Autodesk Inventor part; units mm, degrees
ref_plane "YZ Plane" through (0, 0, 0) normal (1, 0, 0) x (0, 1, 0)
ref_plane "XZ Plane" through (0, 0, 0) normal (0, 1, 0) x (-1, 0, 0)
ref_plane "XY Plane" through (0, 0, 0) normal (0, 0, 1) x (1, 0, 0)
sketch "Sketch1" plane through (0, 0, 0) normal (0, 1, 0) x (-1, 0, 0)
  line L0 (20.5, 16.2) -> (-20.5, 16.2)
  line L1 (-20.5, 16.2) -> (-20.5, -16.2)
  line L2 (-20.5, -16.2) -> (20.5, -16.2)
  line L3 (20.5, -16.2) -> (20.5, 16.2)
  point P0 (0, 0)
  dimension "d0" = 41
  dimension "d1" = 32.4
extrude "Extrusion1" add sketch "Sketch1" along normal blind 3
sketch "Sketch3" plane through (0, 3, 0) normal (0, 1, 0) x (1, 0, 0)
  line L0 (-20.5, -16.2) -> (20.5, -16.2)
  line L1 (-20.5, 16.2) -> (-20.5, -16.2)
  line L2 (20.5, -16.2) -> (-20.5, -16.2)
  line L3 (-20.5, -16.2) -> (-20.5, -13.2)
  line L4 (-20.5, -13.2) -> (20.5, -13.2)
  line L5 (20.5, -13.2) -> (20.5, -16.2)
  line L6 (20.5, 16.2) -> (-20.5, 16.2)
  line L7 (20.5, 16.2) -> (-20.5, 16.2)
  line L8 (-20.5, 16.2) -> (-20.5, 13.2)
  line L9 (-20.5, 13.2) -> (20.5, 13.2)
  line L10 (20.5, 13.2) -> (20.5, 16.2)
  point P0 (0, 0)
  dimension "d8" = 3
  dimension "d9" = 3
extrude "Extrusion3" add sketch "Sketch3" along normal blind 25.4
sketch "Sketch4" plane through (20.5, 0, -16.2) normal (0, 0, -1) x (-1, 0, 0)
  line L0 (41, 3) -> (0, 3)
  line L1 (0, 28.4) -> (41, 28.4)
  line L2 (0, 3) -> (21.5, 3)
  line L3 (21.5, 3) -> (21.5, 28.4)
  line L4 (21.5, 28.4) -> (0, 28.4)
  line L5 (0, 28.4) -> (0, 3)
  point P0 (20.5, 0)
  dimension "d12" = 21.5
extrude "Extrusion4" cut sketch "Sketch4" against normal blind 3
sketch "Sketch5" plane through (-20.5, 0, 16.2) normal (0, 0, 1) x (1, 0, 0)
  line L0 (41, 28.4) -> (0, 28.4)
  line L1 (19.5, 3) -> (41, 3)
  line L2 (0, 28.4) -> (21.5, 28.4)
  line L3 (21.5, 28.4) -> (21.5, 3)
  line L4 (21.5, 3) -> (0, 3)
  line L5 (0, 3) -> (0, 28.4)
  point P0 (20.5, 0)
  dimension "d15" = 21.5
extrude "Extrusion5" cut sketch "Sketch5" against normal blind 3
sketch "Sketch6" plane through (0, 3, 0) normal (0, 1, 0) x (1, 0, 0)
  circle A0 centre (13, 0) radius 4.25
  circle A1 centre (-13, 0) radius 4.25
  line L0 (20.5, -13.2) -> (20.5, 16.2)
  line L1 (-20.5, 13.2) -> (-20.5, -16.2)
  point P0 (0, 0)
  dimension "d20" = 8.5
  dimension "d21" = 8.5
  dimension "d54" = 7.5
  dimension "d65" = 26
  dimension "d66" = 7.5
extrude "Extrusion6" add sketch "Sketch6" along normal blind 3
sketch "Sketch7" plane through (0, 0, 0) normal (0, -1, 0) x (1, 0, 0)
  circle A0 centre (-13, 0) radius 4.25
  circle A1 centre (-13, 0) radius 2
  circle A2 centre (13, 0) radius 4.25
  circle A3 centre (13, 0) radius 2
  point P0 (0, 0)
  dimension "d24" = 4
  dimension "d25" = 4
extrude "Extrusion7" cut sketch "Sketch7" against normal blind 6 contours A1 | A3
sketch "Sketch8" plane through (0, 0, 0) normal (0, -1, 0) x (1, 0, 0)
  circle A0 centre (-13, 0) radius 2
  circle A1 centre (-13, 0) radius 3
  circle A2 centre (13, 0) radius 2
  circle A3 centre (13, 0) radius 3
  point P0 (0, 0)
  dimension "d28" = 6
  dimension "d29" = 6
extrude "Extrusion8" cut sketch "Sketch8" against normal blind 3 contours A0 | A1 | A2 | A3
sketch "Sketch14" plane through (-20.5, 0, 16.2) normal (0, 0, 1) x (1, 0, 0)
  point P0 (20.5, 0)
sketch "Sketch15" plane through (20.5, 0, -16.2) normal (0, 0, -1) x (-1, 0, 0)
  line L0 (0, 0) -> (0, 3)
  line L1 (41, 0) -> (41, 28.4)
  line L2 (0, 0) -> (41, 0)
  line L3 (41, 0) -> (41, 14)
  line L4 (41, 14) -> (0, 14)
  line L5 (0, 14) -> (0, 0)
  line L6 (21.5, 28.4) -> (41, 28.4)
  line L7 (41, 14) -> (37, 14)
  line L8 (37, 14) -> (37, 28.4)
  line L9 (37, 28.4) -> (41, 28.4)
  line L10 (41, 28.4) -> (41, 14)
  line L11 (21.5, 3) -> (21.5, 28.4)
  line L12 (21.5, 14) -> (25.5, 14)
  line L13 (25.5, 14) -> (25.5, 28.4)
  line L14 (25.5, 28.4) -> (21.5, 28.4)
  line L15 (21.5, 28.4) -> (21.5, 14)
  point P0 (20.5, 0)
  dimension "d67" = 14
  dimension "d68" = 4
  dimension "d69" = 4
extrude "Extrusion14" add sketch "Sketch15" along normal blind 4 contours L0 L5 L4 L1 L2 | L4 L8 L6 L1 | L11 L6 L13 L4
sketch "Sketch16" plane through (20.5, 0, -20.2) normal (0, 0, -1) x (-1, 0, 0)
  line L0 (21.5, 14) -> (0, 14)
  line L1 (41, 3) -> (41, 28.4)
  line L2 (0, 14) -> (41, 14)
  line L3 (41, 14) -> (41, 10)
  line L4 (41, 10) -> (0, 10)
  line L5 (0, 10) -> (0, 14)
  point P0 (20.5, 0)
  point P1 (41, 14)
  dimension "d72" = 4
extrude "Extrusion15" add sketch "Sketch16" along normal blind 42.3
sketch "Sketch17" plane through (-1, 14, -16.2) normal (0, 1, 0) x (1, 0, 0)
  circle A0 centre (16.5, 40.65) radius 4
  circle A1 centre (-14.5, 40.65) radius 4
  circle A2 centre (-14.5, 9.65) radius 4
  circle A3 centre (16.5, 9.65) radius 4
  point P0 (1, -16.2)
  dimension "d76" = 8
  dimension "d77" = 8
  dimension "d78" = 8
  dimension "d79" = 8
extrude "Extrusion16" add sketch "Sketch17" along normal blind 2
sketch "Sketch18" plane through (-1, 14, -16.2) normal (0, 1, 0) x (1, 0, 0)
  circle A0 centre (1, 25.15) radius 12.5
  circle A1 centre (-14.5, 40.65) radius 4
  circle A2 centre (-14.5, 40.65) radius 2
  circle A3 centre (-14.5, 9.65) radius 4
  circle A4 centre (-14.5, 9.65) radius 2
  circle A5 centre (16.5, 9.65) radius 4
  circle A6 centre (16.5, 9.65) radius 2
  circle A7 centre (16.5, 40.65) radius 4
  circle A8 centre (16.5, 40.65) radius 2
  point P0 (1, -16.2)
  dimension "d82" = 25
  dimension "d83" = 4
  dimension "d84" = 4
  dimension "d85" = 4
  dimension "d86" = 4
extrude "Extrusion17" cut sketch "Sketch18" along normal mid plane 10 contours A0 | A2 | A4 | A6 | A8
sketch "Sketch19" plane through (15.5, 16, -25.85) normal (0, 1, 0) x (1, 0, 0)
  circle A0 centre (-31, 0) radius 2
  circle A1 centre (-31, 0) radius 3
  circle A2 centre (0, 0) radius 2
  circle A3 centre (0, 0) radius 3
  circle A4 centre (0, 31) radius 2
  circle A5 centre (0, 31) radius 3
  circle A6 centre (-31, 31) radius 2
  circle A7 centre (-31, 31) radius 3
  point P0 (-15.5, -25.85)
  dimension "d89" = 6
  dimension "d90" = 6
  dimension "d91" = 6
  dimension "d92" = 6
extrude "Extrusion18" cut sketch "Sketch19" against normal blind 1.5 contours A0 | A1 | A2 | A3 | A4 | A5 | A6 | A7
sketch "Sketch20" plane through (20.5, 0, 16.2) normal (1, 0, 0) x (0, 0, -1)
  line L0 (36.4, 14) -> (78.7, 14)
  line L1 (78.7, 14) -> (36.4, 14)
  line L2 (36.4, 14) -> (36.4, 10)
  line L3 (36.4, 10) -> (78.7, 10)
  line L4 (78.7, 10) -> (78.7, 14)
  line L5 (32.4, 14) -> (32.4, 3)
  line L6 (36.4, 0) -> (36.4, 10)
  line L7 (32.4, 14) -> (36.4, 14)
  line L8 (36.4, 14) -> (36.4, 0)
  line L9 (36.4, 0) -> (32.4, 0)
  line L10 (32.4, 0) -> (32.4, 14)
  point P0 (16.2, 0)
extrude "Extrusion19" add sketch "Sketch20" along normal blind 5
sketch "Sketch21" plane through (-20.5, 0, 16.2) normal (-1, 0, 0) x (0, 0, 1)
  line L0 (-78.7, 14) -> (-32.4, 14)
  line L1 (-36.4, 10) -> (-78.7, 10)
  line L2 (-78.7, 14) -> (-36.4, 14)
  line L3 (-36.4, 14) -> (-36.4, 10)
  line L4 (-36.4, 10) -> (-78.7, 10)
  line L5 (-78.7, 10) -> (-78.7, 14)
  line L6 (0, 0) -> (-36.4, 0)
  line L7 (-32.4, 0) -> (-36.4, 0)
  line L8 (-36.4, 0) -> (-36.4, 14)
  line L9 (-36.4, 14) -> (-32.4, 14)
  line L10 (-32.4, 14) -> (-32.4, 0)
  point P0 (-16.2, 0)
extrude "Extrusion20" add sketch "Sketch21" along normal blind 5
sketch "Sketch22" plane through (25.5, 10, -62.5) normal (0, -1, 0) x (1, 0, 0)
  line L0 (0, 0) -> (0, 46.3)
  line L1 (-51, 42.3) -> (0, 42.3)
  line L2 (0, 0) -> (-4, 0)
  line L3 (-4, 0) -> (-4, 42.3)
  line L4 (-4, 42.3) -> (0, 42.3)
  line L5 (0, 42.3) -> (0, 0)
  line L6 (-51, 46.3) -> (-51, 0)
  line L7 (-51, 0) -> (-47, 0)
  line L8 (-47, 0) -> (-47, 42.3)
  line L9 (-47, 42.3) -> (-51, 42.3)
  line L10 (-51, 42.3) -> (-51, 0)
  point P0 (-25.5, 62.5)
  dimension "d99" = 4
  dimension "d100" = 4
extrude "Extrusion21" add sketch "Sketch22" along normal blind 10
sketch "Sketch23" plane through (25.5, 0, 16.2) normal (1, 0, 0) x (0, 0, -1)
  line L0 (36.4, 10) -> (78.7, 10)
  line L1 (36.4, 10) -> (36.4, 0)
  line L2 (78.7, 10) -> (36.4, 0)
  line L3 (36.4, 0) -> (78.7, 0)
  line L4 (78.7, 0) -> (78.7, 10)
  point P0 (16.2, 0)
extrude "Extrusion22" cut sketch "Sketch23" against normal blind 60 contours L4 L3 L2
sketch "Sketch24" plane through (-1, 3, -13.2) normal (1, 0, 0) x (0, 0, -1)
  line L0 (7, 25.4) -> (7, 11)
  line L1 (3, 25.4) -> (3, 11)
  line L2 (7, 11) -> (3, 25.4)
  line L3 (0, 25.4) -> (7, 25.4)
  line L4 (3, 25.4) -> (7, 25.4)
  line L5 (7, 25.4) -> (7, 11)
  point P0 (-13.2, -3)
extrude "Extrusion23" cut sketch "Sketch24" against normal blind 60
sketch "Sketch25" plane through (25.5, 0, 16.2) normal (1, 0, 0) x (0, 0, -1)
  line L0 (32.4, 14) -> (32.4, 28.4)
  line L1 (32.4, 14) -> (33.4, 14)
  line L2 (33.4, 14) -> (33.4, 3)
  line L3 (33.4, 3) -> (32.4, 3)
  line L4 (32.4, 3) -> (32.4, 14)
  point P0 (16.2, 0)
  dimension "d107" = 1
extrude "Extrusion24" cut sketch "Sketch25" against normal blind 26.5
sketch "Sketch26" plane through (25.5, 0, 16.2) normal (1, 0, 0) x (0, 0, -1)
  line L0 (33.4, 3) -> (32.4, 3)
  line L1 (32.4, 0) -> (36.4, 0)
  line L2 (32.4, 3) -> (33.4, 3)
  line L3 (33.4, 3) -> (33.4, 0)
  line L4 (33.4, 0) -> (32.4, 0)
  line L5 (32.4, 0) -> (32.4, 3)
  point P0 (16.2, 0)
  dimension "d110" = 1
extrude "Extrusion25" cut sketch "Sketch26" against normal blind 5
fillet "Fillet2" radius 1 7 edges at (20.5, 14.2, 16.2) (20.5, 0, -0.5) (0, 0, 16.2) (-20.5, 0, 0) (-25.5, 14, -39.35) (0, 14, -62.5) (25.5, 14, -39.85)
properties part number "stepperBracketVertical"
Read the model definition and answer for the solid it produces. Units are mm, in the model's axes. A direction names the side the tool comes from. Give positions to 0.01 mm unless a question says otherwise; leave off trailing zeros. Write each loop counter-clockwise with the first axis right and the second up, starting at its lowest first coordinate (ties: lowest second). Pieces come first, ordered by that corner, then holes. Notation, with made-up numbers: (47, 21.25) - (53, 21.25) arc R23 ccw to (53, 40.25) - close; hole circle Ø2 at (-16, 43.25). An arc over 180 degrees is marked (long way). Use CSV: the item, a comma, the result in double quotes. Start each with the question number.
(1) Find section D-D (y = 26.75). Give the vertices of the cut face in (x, z), plus the area to 3 significant figures.
(2) Determine the mould class of faces 1 (the cylindrical face through (15.109, 15.26, -59.824)), 2 (the flat face through (-23, 7, -16.2)), 3 (the flat face through (20.5, 2.6, 6.3)), 4 (the flat face through (0, 3, 0)) for opening direction Z: +Z half, -Z half, draft (parallel to the pull), parting line (faces both ways), or undercut.
(3) Find section B-B (x = 7.5). Give the vertices of the cut face in (y, z).
(4) For faces 5 (the cylindrical face through (14.85, 15.26, -22.92)), 6 (the cylindrical face through (10, 1, 0)), 7 (the flat face through (25.5, 8, -34)), determine the directions among +Z, -Z, +X, -X, +Y, -Y from which every point of the face is accessible in a straight line to the end or side of a thin tool.
(5) Consider line 1 along Z through (x, y) = (-15.5, 12.05); line 2 along X through (y, z) = (12.65, -56.85); line 3 along Z through (x, y) = (15.5, 12.05). Determine where each line is inside the solid, lowest interval first.
(6) Find section C-C (z = -41.35). Give the vertices of the cut face in (x, y), plus the area to 3 significant figures.
(7) Given P1, Ø15.5, axis at x = 15, y = 20, coming from the -Z side; P2, Ø13.5, axis at x = -11, z = -32.5, coming from the +Y side; P3, Ø4, axis at x = 12, z = -1.5, coming from the +Y side; P4, Ø3, axis at x = 9.5, z = -26, coming from the -Y side, each flat-ended and moving along its own axis, determine where each tip first touches the part or whether it passes through.
(8) Find section A-A (y = 5). Give the vertices of the cut face in (x, z), plus the area to 3 significant figures.
Findings below:
1,outline,"(-20.5, -16.66) - (-16.5, -16.66) - (-16.5, -16.2) - (-5, -16.2) - (-5, -16.66) - (-1, -16.66) - (-1, -13.2) - (-20.5, -13.2) - close; (1, 13.2) - (20.5, 13.2) - (20.5, 15.2) arc R1 ccw to (19.5, 16.2) - (1, 16.2) - close"
1,area,"120 mm2"
2,face 1,"undercut"
2,face 2,"+Z half"
2,face 3,"draft"
2,face 4,"undercut"
3,outline,"(0, -20.2) - (10, -20.2) - (10, -31.35) - (14, -31.35) - (14, -17.2) - (3, -17.2) - (3, 13.2) - (28.4, 13.2) - (28.4, 16.2) - (1, 16.2) arc R1 ccw to (0, 15.2) - close; (10, -62.5) - (13, -62.5) arc R1 ccw to (14, -61.5) - (14, -51.35) - (10, -51.35) - close"
4,face 5,"+Y"
4,face 6,"-Y"
4,face 7,"+Z, -Z, +X, +Y, -Y"
5,line 1,"-62.5 to -58.85, -54.85 to -27.85, -23.85 to -13.2"
5,line 2,"-25.5 to -17.5, -13.5 to 13.5, 17.5 to 25.5"
5,line 3,"-62.5 to -58.85, -54.85 to -27.85, -23.85 to -17.2, 13.2 to 16.2"
6,outline,"(-25.5, 5) - (-21.5, 5) - (-21.5, 10) - (-12.5, 10) - (-12.5, 14) - (-24.5, 14) arc R1 ccw to (-25.5, 13) - close; (12.5, 10) - (21.5, 10) - (21.5, 5) - (25.5, 5) - (25.5, 13) arc R1 ccw to (24.5, 14) - (12.5, 14) - close"
6,area,"144 mm2"
7,P1,"z = -62.5"
7,P2,"y = 16"
7,P3,"y = 6"
7,P4,"y = 10"
8,outline,"(-25.5, -41.35) - (-21.5, -41.35) - (-21.5, -20.2) - (21.5, -20.2) - (21.5, -41.35) - (25.5, -41.35) - (25.5, -17.2) - (-1, -17.2) - (-1, -13.2) - (-20.5, -13.2) - (-20.5, -16.2) - (-25.5, -16.2) - close; circle Ø8.5 at (-13, 0); (1, 13.2) - (20.5, 13.2) - (20.5, 15.2) arc R1 ccw to (19.5, 16.2) - (1, 16.2) - close; circle Ø8.5 at (13, 0); hole circle Ø4 at (-13, 0); hole circle Ø4 at (13, 0)"
8,area,"552 mm2"
